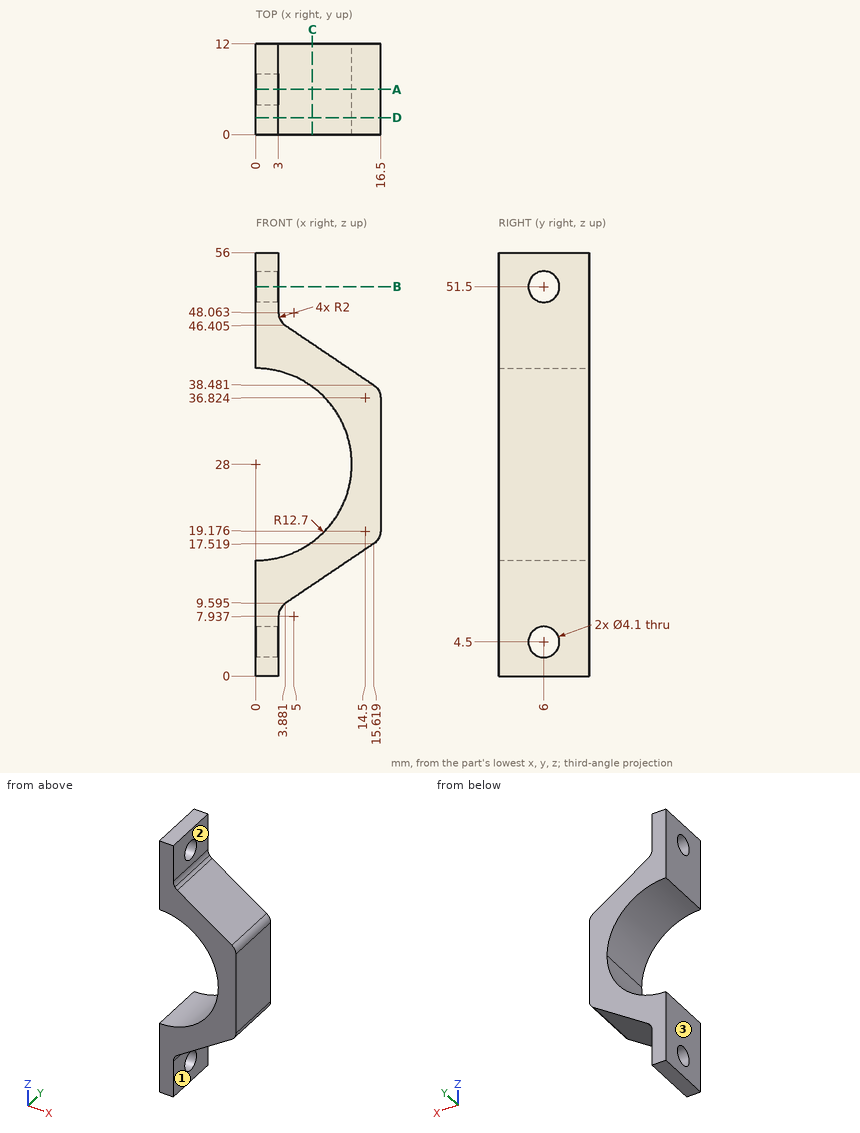
Job drawing, mm, ordinate dimensions from the low corner. One solid piece. A direction names the side the tool comes from. Give positions to 0.01 mm unless a question says otherwise; leave off trailing zeros. Order: outer loops, then holes, each group sorted by start corner. A loop starts at its lowest first (then second) coordinate and runs counter-clockwise, first axis right, second up. Notation, with made-up numbers: (9, -27.5) - (66, -27.5) arc R20 ccw to (66, 3.5) - close; hole circle Ø9 at (82.5, 69.5). An arc over 180 degrees is marked (long way). Return JSON: item names as keys, results as strings.
1) 3-axis set-ups, long thin cutter, end or side, ignore diameter. For the marked faces 1, 2 and 3: which of +Z, -Z, +X, -X, +Y, -Y reach the whole face in a straight line?
Geometry says:
{"face 1": "-Z, +X, +Y, -Y", "face 2": "+Z, +X, +Y, -Y", "face 3": "+Z, -Z, -X, +Y, -Y"}
2) Flat gauge pins, fed straight in: P1, Ø6, axis at y = 5.5, z = 16.5, coming from the +X side; P2, Ø3, axis at x = 6, y = 4.5, coming from the -Z side; P3, Ø3, axis at x = 12, y = 10.5, coming from the -Z side; P4, Ø4.5, axis at y = 6, z = 51.5, coming from the +X side. Where does each tip first touch, or does it go through?
Geometry says:
{"P1": "x = 16.5", "P2": "z = 10.01", "P3": "z = 14.06", "P4": "x = 3"}
3) Cut at B-B, the plane z = 51.5. Give the cut face in (x, y).
Geometry says:
{"outline": "(0, 0) - (3, 0) - (3, 3.95) - (0, 3.95) - close; (0, 8.05) - (3, 8.05) - (3, 12) - (0, 12) - close"}
4) Cut at A-A, the plane y = 6. Count the separate pieces of the cut face and the enclosed holes in it, plus the area to 3 significant figures.
Geometry says:
{"separate pieces": "3", "enclosed holes": "0", "area": "280 mm²"}
5) Cut at C-C, the plane x = 7.5. Give the cut face in (y, z), plus the area to 3 significant figures.
Geometry says:
{"outline": "(0, 12.04) - (12, 12.04) - (12, 17.75) - (0, 17.75) - close; (0, 38.25) - (12, 38.25) - (12, 43.96) - (0, 43.96) - close", "area": "137 mm²"}
6) Probe line 1 (Y direction, x = 0.9, z = 51.5); line 2 (X direction, y = 4.5, z = 6); line 3 (Z direction, x = 9, y = 6). List the from-to ranges inside material, lowest first. Write a range as from..to.
Geometry says:
{"line 1": "0..3.95, 8.05..12", "line 2": "0..3", "line 3": "13.05..19.04, 36.96..42.95"}
7) Cut at D-D, the plane y = 2.25. Give the cut face in (x, z) (1 decimal).
Geometry says:
{"outline": "(0, 0) - (3, 0) - (3, 7.9) arc R2 cw to (3.9, 9.6) - (15.6, 17.5) arc R2 ccw to (16.5, 19.2) - (16.5, 36.8) arc R2 ccw to (15.6, 38.5) - (3.9, 46.4) arc R2 cw to (3, 48.1) - (3, 56) - (0, 56) - (0, 40.7) arc R12.7 cw to (0, 15.3) - close"}
